Input: part model. Units: mm. Frame: model coordinates. Face numbers are marked on the shaded views. A direction names the side the tool comes from. Coordinates: 2 decimals unless noted, no trailing zeros. Write each loop counter-clockwise with the first axis right and the second up, starting at its lowest first coordinate (ties: lowest second). Pieces come first, ordered by that corner, then holes. Notation, with made-up numbers: (23, 50.5) - (28, 50.5) arc R23 ccw to (28, 75.5) - close; hole circle Ø7 at (-13.75, 7.25). An arc over 180 degrees is marked (long way). Put each result on its own line as item: value. Start each with the question number.
1. Cut plane B-B, the plane y = 4. Return loops of the section in (x, z), and give its area (4 significant figures).
2. Access query for the marked faces 1 and 2. Directions: +Z, -Z, +X, -X, +Y, -Y. A direction counts if a zero-diameter tool reaches every point of the face in a straight line with its end or side. Return the directions, or none.
3. Line query: line 1 (Y direction, x = 8.5, z = 7.75); line 2 (Y direction, x = 2, z = 9.25); line 3 (Y direction, x = 2.75, z = 7). Output: solid intervals per line, ascending.
4. Cut plane C-C, the plane y = -26. Return loops of the section in (x, z).
5. Pin query (flat end, axial travel): pin 1 (3 mm diameter, centred on x = 10, z = 9.5, fed in from +Y); pin 2 (2 mm diameter, centred on x = 10.5, z = 10, fed in from +Y); pin 3 (0.5 mm diameter, centred on x = 5.5, z = 8, fed in from -Y). Return the tip coordinate at first contact, or that it passes through.
from build123d import *

# Parameters (mm, degrees)
F1_DEPTH = 15
F2_SIZE  = 3
F3_R     = 4.99999


# Not quite as in the source:
# - a fillet or chamfer is up to 0.001 mm smaller than in the source, because OpenCascade refuses the exact size


with BuildPart() as f1:
    # F0 (on Right) → F1 (new body)
    with BuildSketch(Plane.YZ):
        Polygon((13.5, 7.5), (17.5, 7.5), (18.5, 7.5), (18.5, 11.5), (13.5, 11.5), align=None)
        Polygon((-17.5, 5), (17.5, 5), (17.5, 7.5), (13.5, 7.5), (-13.5, 7.5), (-17.5, 7.5), align=None)
        Polygon((90, 0), (90, 5), (17.5, 5), (-17.5, 5), (-90, 5), (-90, 0), align=None)
        Polygon((-18.5, 7.5), (-17.5, 7.5), (-13.5, 7.5), (-13.5, 11.5), (-18.5, 11.5), align=None)
    extrude(amount=F1_DEPTH)

    # F2
    f2_edges = [f1.edges().sort_by_distance(p)[0] for p in [
        (7.5, -18.5, 11.5),
        (7.5, 18.5, 11.5),
    ]]
    chamfer(f2_edges, length=F2_SIZE)

    # F3 (radius 5 in the source; OpenCascade refuses exactly that, so slightly less here)
    f3_edges = [f1.edges().sort_by_distance(p)[0] for p in [
        (7.5, 90, 5),
        (7.5, -90, 5),
    ]]
    fillet(f3_edges, radius=F3_R)


solid = f1.part
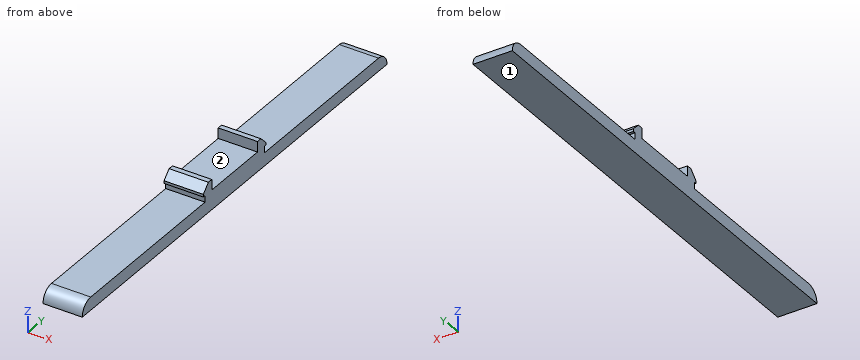
Report:
1. outline: (0, 0) - (15, 0) - (15, 7.5) - (0, 7.5) - close
1. area: 112.5 mm^2
2. face 1: -Z, +X, -X, +Y, -Y
2. face 2: +Z, +X, -X
3. line 1: y = -18.5 to -13.5, 13.5 to 18.5
3. line 2: y = -17.75 to -13.5, 13.5 to 17.75
3. line 3: y = -17.5 to 17.5
4. outline: (0, 0) - (15, 0) - (15, 5) - (0, 5) - close
5. pin 1: stops at y = 18.5
5. pin 2: stops at y = 18
5. pin 3: stops at y = -18.5
